from build123d import *

# Parameters (mm, degrees)
SKETCH1_W                                            = 63.5
SKETCH1_H                                            = 63.5
SKETCH1_R                                            = 3
BOSS_EXTRUDE1_DEPTH                                  = 292.1
FILLET1_R                                            = 2.54
SHELL1_START                                         = -292.1
SHELL1_DEPTH                                         = 584.2
SKETCH3_W                                            = 63.665273771
SKETCH3_H                                            = 31.75
CUT_EXTRUDE2_DEPTH                                   = 586.923002621
CSK_FOR_M6_HEX_SOCKET_COUNTERSUNK_HEAD_S_D           = 6.4
CSK_FOR_M6_HEX_SOCKET_COUNTERSUNK_HEAD_S_CSINK_D     = 13.5
CSK_FOR_M6_HEX_SOCKET_COUNTERSUNK_HEAD_S_CSINK_ANGLE = 90
M6_CLEARANCE_HOLE1_D                                 = 6.6
M6_CLEARANCE_HOLE1_DEPTH                             = 2.54


# Read off the part's stored shape, not the designer's step: Shell1
with BuildPart() as part:
    # Sketch1 → Boss-Extrude1 (new, symmetric)
    with BuildSketch(Plane.XY):
        Rectangle(SKETCH1_W, SKETCH1_H)
        with Locations((-25.4, 25.4)):
            Circle(SKETCH1_R, mode=Mode.SUBTRACT)
        with Locations(Location((25.4, -25.4, 0), (0, 0, 180))):
            Circle(SKETCH1_R, mode=Mode.SUBTRACT)
        with Locations(Location((-25.4, -25.4, 0), (0, 0, 180))):
            Circle(SKETCH1_R, mode=Mode.SUBTRACT)
        with Locations(Location((25.4, 25.4, 0), (0, 0, 180))):
            Circle(SKETCH1_R, mode=Mode.SUBTRACT)
    extrude(amount=BOSS_EXTRUDE1_DEPTH, both=True)

    # Fillet1
    fillet1_edges = [part.edges().sort_by_distance(p)[0] for p in [
        (31.75, -31.75, 0),
        (-31.75, -31.75, 0),
        (-31.75, 31.75, 0),
        (31.75, 31.75, 0),
    ]]
    fillet(fillet1_edges, radius=FILLET1_R)

    # Shell1 outline → Shell1 (cut)
    with BuildSketch(Plane.XY.offset(SHELL1_START)):
        with BuildLine():
            Line((29.21, -21.378122329), (29.21, 21.378122329))
            ThreePointArc((29.21, 21.378122329), (21.482628432, 21.482628432), (21.378122329, 29.21))
            Line((21.378122329, 29.21), (-21.378122329, 29.21))
            ThreePointArc((-21.378122329, 29.21), (-21.482628432, 21.482628432), (-29.21, 21.378122329))
            Line((-29.21, 21.378122329), (-29.21, -21.378122329))
            ThreePointArc((-29.21, -21.378122329), (-21.482628432, -21.482628432), (-21.378122329, -29.21))
            Line((-21.378122329, -29.21), (21.378122329, -29.21))
            ThreePointArc((21.378122329, -29.21), (21.482628432, -21.482628432), (29.21, -21.378122329))
        make_face()
    extrude(amount=SHELL1_DEPTH, mode=Mode.SUBTRACT)

    # Sketch3 → Cut-Extrude2 (cut, through all)
    with BuildSketch(Plane.XY.offset(292.1)):
        with Locations((0.082636885, -16.003852467)):
            Rectangle(SKETCH3_W, SKETCH3_H)
    extrude(amount=-CUT_EXTRUDE2_DEPTH, mode=Mode.SUBTRACT)

    # CSK for M6 Hex Socket Countersunk Head Screw1 (through all)
    with Locations(Plane(origin=(0, 31.75, 0), x_dir=(1, 0, 0), z_dir=(0, 1, 0))):
        with Locations((0, 203.2), (0, -203.2)):
            CounterSinkHole(CSK_FOR_M6_HEX_SOCKET_COUNTERSUNK_HEAD_S_D / 2, CSK_FOR_M6_HEX_SOCKET_COUNTERSUNK_HEAD_S_CSINK_D / 2, counter_sink_angle=CSK_FOR_M6_HEX_SOCKET_COUNTERSUNK_HEAD_S_CSINK_ANGLE)

    # M6 Clearance Hole1
    with Locations(Plane(origin=(31.75, 0, 0), x_dir=(0, 0, -1), z_dir=(1, 0, 0))):
        with Locations((63.5, 11.811849331), (-63.5, 11.811849331)):
            Hole(M6_CLEARANCE_HOLE1_D / 2, depth=M6_CLEARANCE_HOLE1_DEPTH)


solid = part.part
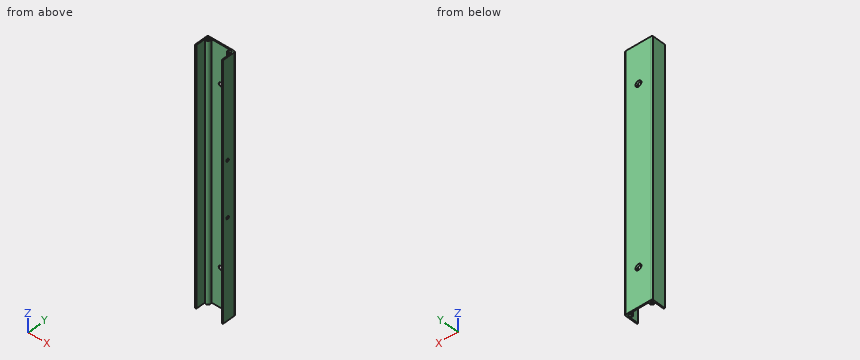
Check sheet for the modelled part. Datum: model origin and axes. Units: mm. Coordinates: 2 decimals unless noted, no trailing zeros. Loops run counter-clockwise (first coordinate to the right, second up) from the corner with the lowest first, then second, coordinate; pieces in that order, holes last. Notation, with made-up numbers: (75.5, -4) -> (113.5, -4) arc R32 cw to (113.5, 26) -> close; hole circle Ø2 at (20.5, 71). An arc over 180 degrees is marked (long way). Answer in a Markdown table with one row per item.
1. Go/stop test with flat-tipped pins: pin 1 (9.5 mm diameter, centred on x = 25.4, y = 25.4, fed in from +Z); pin 2 (3 mm diameter, centred on x = -8, z = -15.5, fed in from -Y). Record where each tip stops, or that it passes through.
Check values:
| item | result |
|---|---|
| pin 1 | stops at z = 292.1 |
| pin 2 | stops at y = 29.21 |
2. Sectioned sample at A-A, the plane z = 203.2. Record the boundary of the cut face in (x, y).
Check values:
| item | result |
|---|---|
| outline | (-31.75, -0.13) -> (-29.21, -0.13) -> (-29.21, 21.38) arc R5.54 ccw to (-21.38, 29.21) -> (-4.21, 29.21) -> (-6.75, 31.75) -> (-29.21, 31.75) arc R2.54 ccw to (-31.75, 29.21) -> close; (4.21, 29.21) -> (21.38, 29.21) arc R5.54 ccw to (29.21, 21.38) -> (29.21, -0.13) -> (31.75, -0.13) -> (31.75, 29.21) arc R2.54 ccw to (29.21, 31.75) -> (6.75, 31.75) -> close; hole circle Ø6 at (-25.4, 25.4); hole circle Ø6 at (25.4, 25.4) |
3. Material ranges on line 1 along X through (y, z) = (25, 11); line 2 along Y through (x, z) = (-25, 8); line 3 along X through (y, z) = (9, -171.5), recorded low to high. Write a range as [from, to].
Check values:
| item | result |
|---|---|
| line 1 | x = [-31.75, -28.37], [-22.43, -19.87], [19.87, 22.43], [28.37, 31.75] |
| line 2 | y = [19.87, 22.43], [28.37, 31.75] |
| line 3 | x = [-31.75, -29.21], [29.21, 31.75] |
4. Sectioned sample at B-B, the plane z = -5.5. Record the boundary of the cut face in (x, y).
Check values:
| item | result |
|---|---|
| outline | (-31.75, -0.13) -> (-29.21, -0.13) -> (-29.21, 21.38) arc R5.54 ccw to (-21.38, 29.21) -> (21.38, 29.21) arc R5.54 ccw to (29.21, 21.38) -> (29.21, -0.13) -> (31.75, -0.13) -> (31.75, 29.21) arc R2.54 ccw to (29.21, 31.75) -> (-29.21, 31.75) arc R2.54 ccw to (-31.75, 29.21) -> close; hole circle Ø6 at (-25.4, 25.4); hole circle Ø6 at (25.4, 25.4) |
5. Sectioned sample at C-C, the plane x = 12. Record the boundary of the cut face in (y, z), then the cut area to 3 significant figures.
Check values:
| item | result |
|---|---|
| outline | (29.21, -292.1) -> (31.75, -292.1) -> (31.75, 292.1) -> (29.21, 292.1) -> close |
| area | 1,480 mm2 |
